```python
from build123d import *

# Parameters (mm, degrees)
BOSS_EXTRUDE1_DEPTH             = 36.4
CUT_EXTRUDE1_START              = -4
SKETCH2_OUTSIDE_W               = 73.904
SKETCH2_OUTSIDE_H               = 27.904
CUT_EXTRUDE1_DEPTH              = 28.4
CHAMFER1_SIZE                   = 2
CHAMFER1_SIZE2                  = 3
TAP_DRILL_FOR_M2X0_4_TAP1_D     = 1.6
TAP_DRILL_FOR_M2X0_4_TAP1_DEPTH = 4


with BuildPart() as part:
    # Sketch1 → Boss-Extrude1 (new body)
    with BuildSketch(Plane.XY):
        Polygon((0, 12), (58, 12), (58, 8), (52.95, 8), (52.95, 0), (5.05, 0), (5.05, 8), (0, 8), align=None)
        with BuildLine():
            Line((12, 8), (46, 8))
            ThreePointArc((46, 8), (48, 6), (46, 4))
            Line((46, 4), (12, 4))
            ThreePointArc((12, 4), (10, 6), (12, 8))
        make_face(mode=Mode.SUBTRACT)
    extrude(amount=BOSS_EXTRUDE1_DEPTH)

    # Sketch2 outside → Cut-Extrude1 (cut)
    with BuildSketch(Plane.XY.offset(36.4).offset(CUT_EXTRUDE1_START)):
        with Locations((29, 6)):
            Rectangle(SKETCH2_OUTSIDE_W, SKETCH2_OUTSIDE_H)
        with BuildLine():
            Line((10.25, 8.75), (47.75, 8.75))
            ThreePointArc((47.75, 8.75), (48.457106781, 8.457106781), (48.75, 7.75))
            Line((48.75, 7.75), (48.75, 4.25))
            ThreePointArc((48.75, 4.25), (48.457106781, 3.542893219), (47.75, 3.25))
            Line((47.75, 3.25), (10.25, 3.25))
            ThreePointArc((10.25, 3.25), (9.542893219, 3.542893219), (9.25, 4.25))
            Line((9.25, 4.25), (9.25, 7.75))
            ThreePointArc((9.25, 7.75), (9.542893219, 8.457106781), (10.25, 8.75))
        make_face(mode=Mode.SUBTRACT)
    extrude(amount=-CUT_EXTRUDE1_DEPTH, mode=Mode.SUBTRACT)

    # Chamfer1
    chamfer1_edges = [part.edges().sort_by_distance(p)[0] for p in [
        (29, 0, 36.4),
    ]]
    chamfer1_side = [part.faces().sort_by_distance(p)[0] for p in [
        (29, 0, 34.4),
    ]]
    chamfer(chamfer1_edges, length=CHAMFER1_SIZE, length2=CHAMFER1_SIZE2, reference=chamfer1_side[0])

    # Tap Drill for M2x0.4 Tap1
    with Locations(Plane(origin=(0, 12, 0), x_dir=(1, 0, 0), z_dir=(0, 1, 0))):
        with Locations((2.5, -2), (55.5, -2), (55.5, -34.4), (2.5, -34.4)):
            Hole(TAP_DRILL_FOR_M2X0_4_TAP1_D / 2, depth=TAP_DRILL_FOR_M2X0_4_TAP1_DEPTH)


solid = part.part
```
Source: CAD feature listing. Evaluate the final solid. Frame: model axes, mm. A direction names the side the tool comes from. Give positions to 0.01 mm unless a question says otherwise; leave off trailing zeros. Write each loop counter-clockwise with the first axis right and the second up, starting at its lowest first coordinate (ties: lowest second). Pieces come first, ordered by that corner, then holes.
1. Section query D-D (y = 6). Return the cut outline in (x, z), then the cut area to 3 significant figures.
2. Section query A-A (x = 13). Return the cut outline in (y, z), then the cut area to 3 significant figures.
3. Material intervals for line 1 along Z through (x, y) = (2.5, 9.4); line 2 along X through (y, z) = (10.2, 2); line 3 along Y through (x, z) = (34, 23.5), sorted ascending.
4. Pull-direction query (Z, two-part tool) for faces 1 (the face through (29, 9, 0)), 2 (the face through (29, 3.25, 18)), 3 (the face through (58, 10, 34)); classes: +Z half, -Z half, draft (parallel to the pull), parting line (faces both ways), or undercut.
5. Section query C-C (z = 6). Return the cut outline in (x, y).
6. First-contact query: pin 1 (1.5 mm diameter, centred on x = 46.5, z = 17, fed in from +Y); pin 2 (1 mm diameter, centred on x = 2.5, z = 2, fed in from -Y); pin 3 (3 mm diameter, centred on x = 56, z = 2.5, fed in from -Y); pin 4 (1.2 mm diameter, centred on y = 6, z = 2.5, fed in from -X). Flat tips, straight axial feed; report the tip coordinate or a pass-through.
7. Section query B-B (y = 10.25). Return the cut outline in (x, z), then the cut area to 3 significant figures.
8. Access query for faces 4 (the face through (29, 8.75, 18)), 5 (the face through (48.75, 6, 18)), 6 (the face through (5.05, 4, 2)). Directions: +Z, -Z, +X, -X, +Y, -Y. A direction counts if a zero-diameter tool reaches every point of the face in a straight line with its end or side. Return the directions, or none.
Output values:
1. outline: (5.05, 0) - (10, 0) - (10, 36.4) - (5.05, 36.4) - (5.05, 32.4) - (9.25, 32.4) - (9.25, 4) - (5.05, 4) - close; (48, 0) - (52.95, 0) - (52.95, 4) - (48.75, 4) - (48.75, 32.4) - (52.95, 32.4) - (52.95, 36.4) - (48, 36.4) - close
1. area: 122 mm2
2. outline: (0, 0) - (4, 0) - (4, 36.4) - (3, 36.4) - (0, 34.4) - (0, 32.4) - (3.25, 32.4) - (3.25, 4) - (0, 4) - close; (8, 0) - (12, 0) - (12, 4) - (8.75, 4) - (8.75, 32.4) - (12, 32.4) - (12, 36.4) - (8, 36.4) - close
2. area: 104 mm2
3. line 1: z = 0 to 1.2, 2.8 to 4, 32.4 to 33.6, 35.2 to 36.4
3. line 2: x = 0 to 1.7, 3.3 to 54.7, 56.3 to 58
3. line 3: y = 3.25 to 4, 8 to 8.75
4. face 1: -Z half
4. face 2: undercut
4. face 3: draft
5. outline: (9.25, 4.25) arc R1 ccw to (10.25, 3.25) - (47.75, 3.25) arc R1 ccw to (48.75, 4.25) - (48.75, 7.75) arc R1 ccw to (47.75, 8.75) - (10.25, 8.75) arc R1 ccw to (9.25, 7.75) - close; hole (12, 4) - (46, 4) arc R2 ccw to (46, 8) - (12, 8) arc R2 ccw to start
6. pin 1: stops at y = 8.75
6. pin 2: passes through
6. pin 3: stops at y = 8
6. pin 4: stops at x = 5.05
7. outline: (0, 0) - (58, 0) - (58, 4) - (0, 4) - close; (0, 32.4) - (58, 32.4) - (58, 36.4) - (0, 36.4) - close; hole circle Ø1.6 at (2.5, 2); hole circle Ø1.6 at (2.5, 34.4); hole circle Ø1.6 at (55.5, 2); hole circle Ø1.6 at (55.5, 34.4)
7. area: 456 mm2
8. face 4: +X, -X, +Y
8. face 5: +X, +Y, -Y
8. face 6: +Z, -Z, -X, -Y
